Geometry check sheet. Reference: the model listing, model coordinates, mm. A direction names the side the tool comes from. Give positions to 0.01 mm unless a question says otherwise; leave off trailing zeros. Loops run counter-clockwise (first coordinate to the right, second up) from the corner with the lowest first, then second, coordinate; pieces in that order, holes last. Notation, with made-up numbers: (-1, -8) -> (25, -8) arc R20 ccw to (25, 11) -> close; hole circle Ø7 at (56.5, 32.5). An arc over 180 degrees is marked (long way). Answer in a Markdown table with one row per item. Add a question column.
```python
from build123d import *

# Parameters (mm, degrees)
F0_R     = 31.75
F0_W     = 43.18
F0_H     = 13.97
F0_H_2   = 3.81
F1_DEPTH = 7.62
F3_DEPTH = 7.62
F4_DEPTH = 76.2
F5_DEPTH = 7.62


with BuildPart() as f1:
    # F0 (on Right) → F1 (new body)
    with BuildSketch(Plane.YZ):
        with BuildLine():
            ThreePointArc((-21.2379042244, -275.0427409069), (-4.5168222767, -258.7284761869), (1.6220957756, -236.1882122133))
            ThreePointArc((1.6220957756, -236.1882122133), (-65.368168198, -197.8771302656), (-64.4179042244, -275.0427409069))
            Line((-64.4179042244, -275.0427409069), (-21.2379042244, -275.0427409069))
        make_face()
        with Locations((-42.8279042244, -236.1882122133)):
            Circle(F0_R, mode=Mode.SUBTRACT)
        with Locations((-42.8279042244, -236.1882122133)):
            Circle(F0_R)
        with Locations((-42.8279042244, -293.4577409069)):
            Rectangle(F0_W, F0_H)
        with BuildLine():
            ThreePointArc((-21.2379042244, -275.0427409069), (-42.8279042244, -280.6382122133), (-64.4179042244, -275.0427409069))
            Line((-64.4179042244, -275.0427409069), (-64.4179042244, -282.6627409069))
            Line((-64.4179042244, -282.6627409069), (-21.2379042244, -282.6627409069))
            Line((-21.2379042244, -282.6627409069), (-21.2379042244, -275.0427409069))
        make_face()
        with Locations((-42.8279042244, -284.5677409069)):
            Rectangle(F0_W, F0_H_2)
        with BuildLine():
            Line((-21.2379042244, -275.0427409069), (-64.4179042244, -275.0427409069))
            ThreePointArc((-64.4179042244, -275.0427409069), (-42.8279042244, -280.6382122133), (-21.2379042244, -275.0427409069))
        make_face()
    extrude(amount=F1_DEPTH)

    # F0 (on Right) → F3 (join)
    with BuildSketch(Plane.YZ):
        with BuildLine():
            ThreePointArc((-21.2379042244, -275.0427409069), (-4.5168222767, -258.7284761869), (1.6220957756, -236.1882122133))
            ThreePointArc((1.6220957756, -236.1882122133), (-65.368168198, -197.8771302656), (-64.4179042244, -275.0427409069))
            Line((-64.4179042244, -275.0427409069), (-21.2379042244, -275.0427409069))
        make_face()
        with Locations((-42.8279042244, -236.1882122133)):
            Circle(F0_R, mode=Mode.SUBTRACT)
    extrude(amount=F3_DEPTH)

    # F2 (on face) → F4 (cut)
    with BuildSketch(Plane.YZ.offset(7.62)):
        with BuildLine():
            Line((-60.6079042244, -276.6458034995), (-60.6079042244, -296.6327409069))
            Line((-60.6079042244, -296.6327409069), (-25.0479042244, -296.6327409069))
            Line((-25.0479042244, -296.6327409069), (-25.0479042244, -276.6458034995))
            ThreePointArc((-25.0479042244, -276.6458034995), (-42.8279042244, -279.8589187517), (-60.6079042244, -276.6458034995))
        make_face()
    extrude(amount=-F4_DEPTH, mode=Mode.SUBTRACT)

    # F0 (on Right) → F5 (join)
    with BuildSketch(Plane.YZ):
        with Locations((-42.8279042244, -284.5677409069)):
            Rectangle(F0_W, F0_H_2)
    extrude(amount=-F5_DEPTH)


solid = f1.part
```
1. Gauge pin test, flat ends, axial feed: pin 1 Ø4 at (x, z) = (3, -290.5) entering from -Y; pin 2 Ø8 at (x, y) = (1, -59) entering from +Z; pin 3 Ø4 at (x, z) = (4.5, -287) entering from +Y. Record the tip position at first contact, or that the pin passes through.
2. Release check for a two-part mould opening along Y. For faces 5 (the face through (4, -43, -296.633)), 6 (the face through (0, -43, -298)), 7 (the face through (3, -21.238, -288)), 8 (the face through (3, -64.418, -288)) record: released by +Y, released by -Y, zero draft, split by the parting line, or undercut.
3. Sectioned sample at C-C (x = -6). Enter the section's corners in (y, z).
4. Access from +Z, -Z, +X, -X, +Y, -Y to the whole of each face (thin tool, end or side, straight path). Record for faces 1 (the face through (-4, -43, -282.663)), 2 (the face through (-4, -43, -286.473)), 3 (the face through (-7.62, -43, -285)), 4 (the face through (0, -43, -285)).
5. Sectioned sample at D-D (y = -52). Enter the section's corners in (x, z), plus the area to 3 significant figures.
6. Material ranges on L1, parallel to X at y = -62, z = -254; L2, parallel to Z at x = -5.25, y = -25.5; L3, parallel to Y at x = -6, z = -284, recorded low to high. Write a range as from..to.
7. Sectioned sample at B-B (x = 1.25). Enter the section's corners in (y, z).
8. Sectioned sample at A-A (y = -30.5). Enter the section's corners in (x, z), plus the area to 3 significant figures.
Response:
| question | item | result |
|---|---|---|
| 1 | pin 1 | stops at y = -64.42 |
| 1 | pin 2 | stops at z = -193.44 |
| 1 | pin 3 | stops at y = -21.24 |
| 2 | face 5 | undercut |
| 2 | face 6 | zero draft |
| 2 | face 7 | released by +Y |
| 2 | face 8 | released by -Y |
| 3 | outline | (-64.42, -286.47) -> (-21.24, -286.47) -> (-21.24, -282.66) -> (-64.42, -282.66) -> close |
| 4 | face 1 | +Z, -X, +Y, -Y |
| 4 | face 2 | -Z, -X, +Y, -Y |
| 4 | face 3 | +Z, -Z, -X, +Y, -Y |
| 4 | face 4 | +X |
| 5 | outline | (-7.62, -286.47) -> (0, -286.47) -> (0, -282.66) -> (-7.62, -282.66) -> close; (0, -300.44) -> (7.62, -300.44) -> (7.62, -296.63) -> (0, -296.63) -> close; (0, -279.02) -> (7.62, -279.02) -> (7.62, -192.69) -> (0, -192.69) -> close |
| 5 | area | 716 mm2 |
| 6 | L1 | x = 0..7.62 |
| 6 | L2 | z = -286.47..-282.66 |
| 6 | L3 | y = -64.42..-21.24 |
| 7 | outline | (-64.42, -300.44) -> (-21.24, -300.44) -> (-21.24, -275.04) arc R44.45 ccw (long way) to (-64.42, -275.04) -> close; hole (-60.61, -296.63) -> (-25.05, -296.63) -> (-25.05, -276.65) arc R50.8 cw to (-60.61, -276.65) -> close |
| 8 | outline | (-7.62, -286.47) -> (0, -286.47) -> (0, -282.66) -> (-7.62, -282.66) -> close; (0, -300.44) -> (7.62, -300.44) -> (7.62, -296.63) -> (0, -296.63) -> close; (0, -278.34) -> (7.62, -278.34) -> (7.62, -193.48) -> (0, -193.48) -> close |
| 8 | area | 705 mm2 |
